Source: three-view drawing plus pictorial views. Frame: mm from the lowest corner of the part. A direction names the side the tool comes from. Give positions to 0.01 mm unless a question says otherwise; leave off trailing zeros. Order: outer loops, then holes, each group sorted by start corner. A loop starts at its lowest first (then second) coordinate and runs counter-clockwise, first axis right, second up.
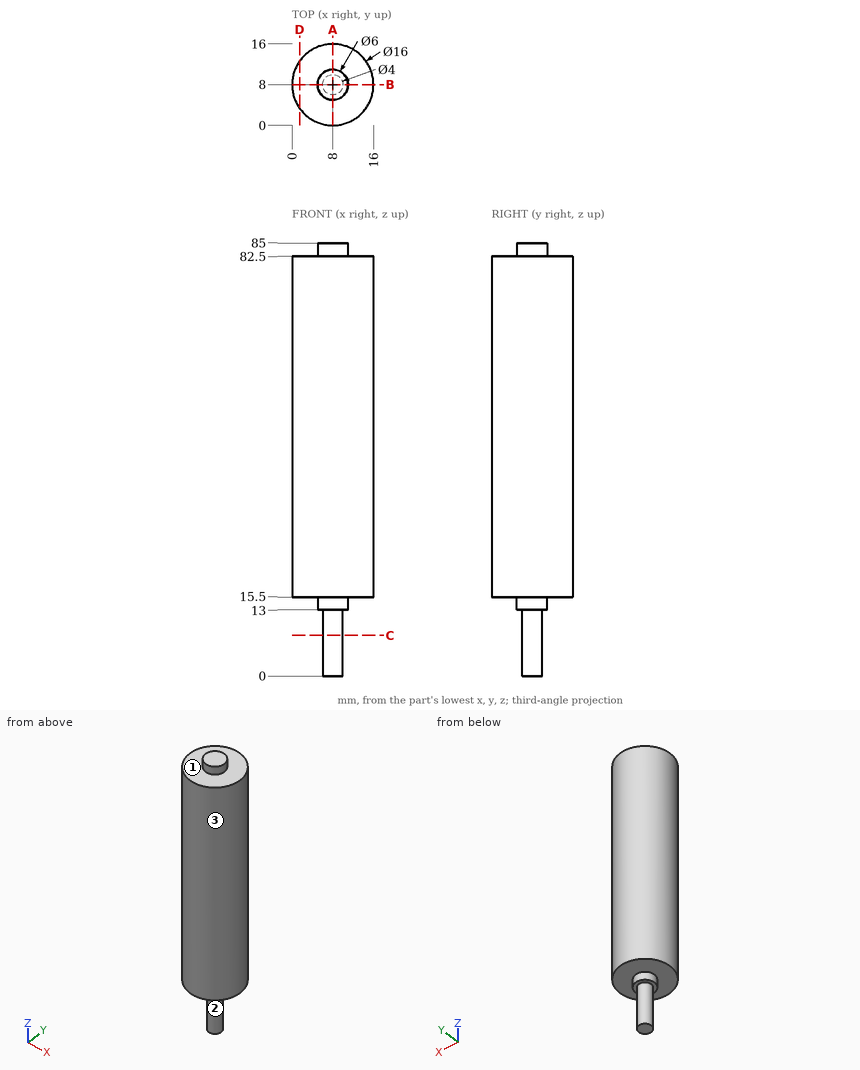
(1) Line query: line 1 along Z through (x, y) = (5.75, 8.75); line 2 along Z through (x, y) = (2.75, 5); line 3 along X through (y, z) = (8.5, 42). Output: solid intervals per line, ascending.
(2) Access query for the marked faces 1, 2 and 3. Directions: +Z, -Z, +X, -X, +Y, -Y. A direction counts if a zero-diameter tool reaches every point of the face in a straight line with its end or side. Return the directions, or none.
(3) Section A-A, the plane x = 8. Return loops of the section in (y, z), plus the area to 3 significant figures.
(4) Section C-C, the plane z = 8. Return loops of the section in (x, y), plus the area to 3 significant figures.
(5) Section D-D, the plane x = 1.5. Return loops of the section in (y, z).
(6) Pin query (flat end, axial travel): pin 1 Ø2 at (x, y) = (9, 6) entering from -Z; pin 2 Ø2 at (x, y) = (9.5, 14) entering from +Z; pin 3 Ø4 at (y, z) = (5.5, 44) entering from +X; pin 4 Ø1.5 at (x, y) = (4.5, 11.5) entering from -Z. Return the tip coordinate at first contact, or that it passes through.
Checks:
1. line 1: z = 13 to 85
1. line 2: z = 15.5 to 82.5
1. line 3: x = 0.02 to 15.98
2. face 1: +Z
2. face 2: -Z
2. face 3: +Z, -Z
3. outline: (0, 15.5) - (5, 15.5) - (5, 13) - (6, 13) - (6, 0) - (10, 0) - (10, 13) - (11, 13) - (11, 15.5) - (16, 15.5) - (16, 82.5) - (11, 82.5) - (11, 85) - (5, 85) - (5, 82.5) - (0, 82.5) - close
3. area: 1,150 mm2
4. outline: circle Ø4 at (8, 8)
4. area: 12.6 mm2
5. outline: (3.34, 15.5) - (12.66, 15.5) - (12.66, 82.5) - (3.34, 82.5) - close
6. pin 1: stops at z = 0
6. pin 2: stops at z = 82.5
6. pin 3: stops at x = 15.98
6. pin 4: stops at z = 15.5
